Autodesk Inventor part; units mm, degrees
ref_plane "作業平面2" through (-121.2214, 0, 2.9367) normal (-0.5592, 0, 0.829) x (0, -1, 0)
ref_plane "YZ Plane" through (0, 0, 0) normal (1, 0, 0) x (0, 1, 0)
ref_plane "XZ Plane" through (0, 0, 0) normal (0, 1, 0) x (-1, 0, 0)
sketch "スケッチ1" plane through (0, 0, 0) normal (0, 1, 0) x (-1, 0, 0)
  arc A0 (41.4452, -14.9694) -> (120.7701, -0.6068) centre (36.8758, 236.5065) ccw
  arc A1 (30.7183, -14.8468) -> (41.4452, -14.9694) centre (38.1525, 166.2425) ccw
  arc A2 (11.0166, -11.3447) -> (30.7183, -14.8468) centre (33.77, 59.49) ccw
  arc A3 (-0.3565, -5.7585) -> (11.0166, -11.3447) centre (24.3575, 30.1875) ccw
  arc A4 (-3.5852, -2.6234) -> (-0.3565, -5.7585) centre (7.25, 5.305) ccw
  arc A5 (-0.7848, 4.3726) -> (-3.5852, -2.6234) centre (0, 0) ccw
  arc A6 (7.6183, 5.1344) -> (-0.7848, 4.3726) centre (7.775, -43.32) ccw
  arc A7 (35.5607, 3.8888) -> (7.6183, 5.1344) centre (8.565, -287.665) ccw
  arc A8 (35.5607, 3.8888) -> (52.6853, 2.3311) centre (526.9475, 5310.875) ccw
  arc A9 (52.6853, 2.3311) -> (84.6244, 0.9905) centre (82.86, 340.0849) ccw
  arc A10 (84.6244, 0.9905) -> (119.8564, 3.2634) centre (83.0725, 299.245) ccw
  arc A11 (120.7701, -0.6068) -> (119.8564, 3.2634) centre (120.103, 1.2786) ccw
  point P0 (0, 0)
extrude "押し出し1" add sketch "スケッチ1" along normal mid plane 250
sketch "スケッチ2" plane through (0, -125, 0) normal (0, -1, 0) x (1, 0, 0)
  circle A0 centre (-85, -5) radius 3
  circle A1 centre (-10, -2) radius 3
  point P0 (0, 0)
extrude "押し出し2" cut sketch "スケッチ2" against normal up to next
ref_plane "作業平面2" through (-121.2214, 0, 2.9367) normal (-0.5592, 0, 0.829) x (0, -1, 0)
ref_plane "作業平面1" through (-146.4564, 100, -7.5667) normal (-0.5592, 0, 0.829) x (0.829, 0, 0.5592)
sketch "スケッチ3" plane through (-121.2214, 0, 2.9367) normal (-0.5592, 0, 0.829) x (0, -1, 0)
  arc A0 (-135, -26.7942) -> (-100, 63.2058) centre (-233.2143, 63.2058) ccw
  line L0 (-100, 63.2058) -> (-100, 73.2058)
  line L1 (-100, 473.2058) -> (-100, 73.2058)
  line L2 (-135, -26.7942) -> (-135, 113.2058)
  line L3 (-135, 113.2058) -> (-100, 113.2058)
  point P0 (0, 98.855)
  dimension "d6" = 140
extrude "押し出し3" cut sketch "スケッチ3" against normal through all
properties part number "subflap_top"
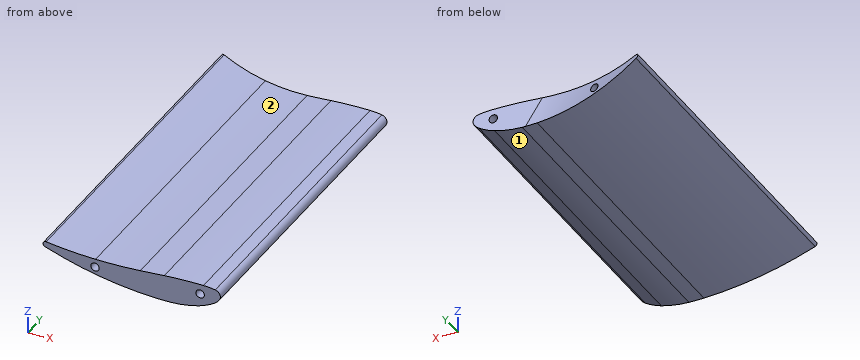
Model file for the job. Use its own axes, mm. Face numbers are marked on the shaded views. A direction names the side the tool comes from. Coordinates: 2 decimals unless noted, no trailing zeros. Loops run counter-clockwise (first coordinate to the right, second up) from the corner with the lowest first, then second, coordinate; pieces in that order, holes last. Notation, with made-up numbers: M 32,87 L 60,87 A21 ccw 60,105 Z; hole C 21.5,14.25 d4. An arc over 180 degrees is marked long. Use CSV: the item, a comma, the result in double quotes. Start each with the question number.
1. Band-saw the part on A-A, the plane y = -89. List the corners of the cut face in (x, z).
2. Tool access for the marked faces 1 and 2: list every direction of +Z, -Z, +X, -X, +Y, -Y with a clear straight run to the whole face (end or side of a thin tool).
3. Flat gauge pins, fed straight in: pin 1 (4 mm diameter, centred on x = -48, y = -10.5, fed in from -Z); pin 2 (12 mm diameter, centred on x = -99.5, y = 52.5, fed in from +Z); pin 3 (2 mm diameter, centred on x = -45.5, z = 2, fed in from +Y); pin 4 (2 mm diameter, centred on x = -100, z = -8.5, fed in from -Y). Where does each tip first touch, or does it go through?
4. Band-saw the part on B-B, the plane x = -26. List the corners of the cut face in (y, z), then the cut area to 3 significant figures.
5. Probe probe 1 along Z at (x, y) = (-10, -48.5); probe 2 along Y at (x, z) = (-5.5, -4); probe 3 along Z at (x, y) = (-12, -8.5). List the from-to ranges inside material, lowest first. Write a range as [from, to].
Entries:
1,outline,"M -120.77,-0.61 A251.51 ccw -41.45,-14.97 A181.22 ccw -30.72,-14.85 A74.4 ccw -11.02,-11.34 A43.63 ccw 0.36,-5.76 A13.42 ccw 3.59,-2.62 A4.44 ccw 0.78,4.37 A48.46 ccw -7.62,5.13 A292.8 ccw -35.56,3.89 A5310.23 cw -52.69,2.33 A339.09 cw -84.62,0.99 A298.26 cw -119.86,3.26 A2 ccw Z; hole C -85,-5 d6; hole C -10,-2 d6"
2,face 1,"-Z, +X, +Y, -Y"
2,face 2,"+Z, +Y, -Y"
3,pin 1,"stops at z = -14.85"
3,pin 2,"stops at z = 1.83"
3,pin 3,"stops at y = 100.01"
3,pin 4,"passes through"
4,outline,"M -125,-14.5 L 100,-14.5 L 100,4.62 L -125,4.62 Z"
4,area,"4,300 mm2"
5,probe 1,"z = [-11, -5], [1, 5.13]"
5,probe 2,"y = [-125, 100]"
5,probe 3,"z = [-11.65, -4.24], [0.24, 5.12]"
